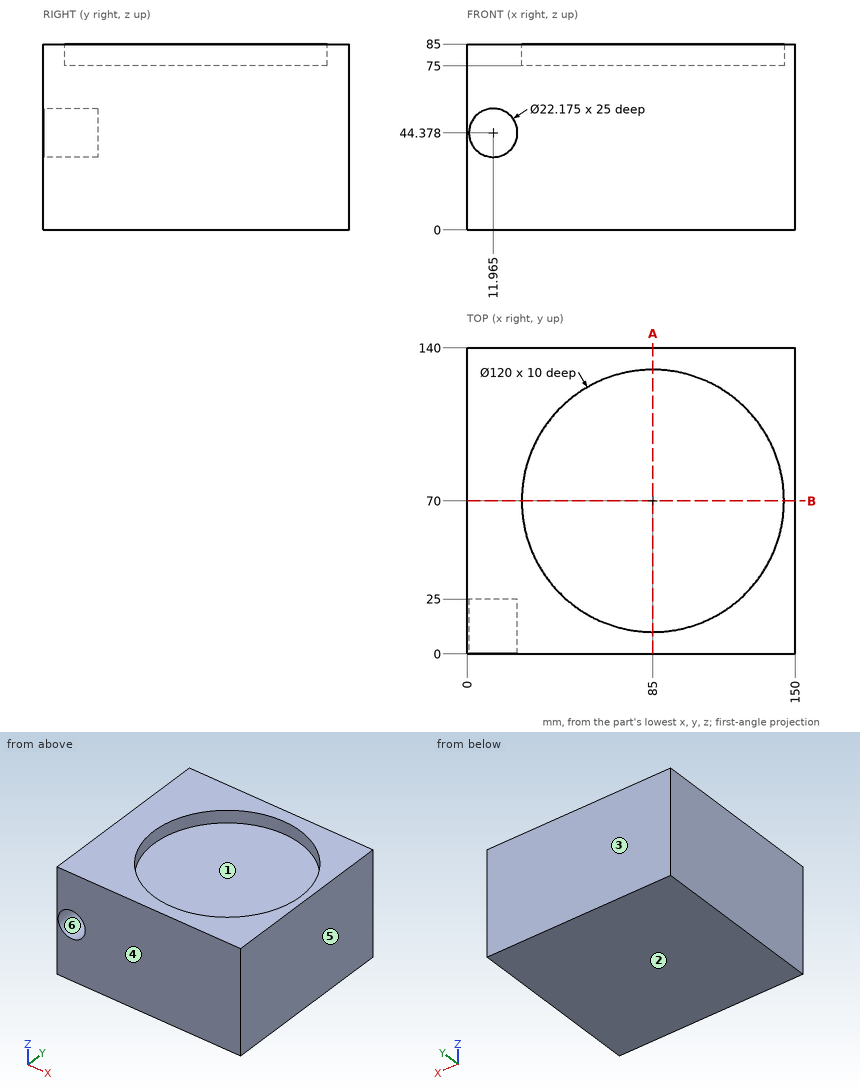
Here's the drawing with two shaded views (mm, measured from the low corner). I have some questions. A direction names the side the tool comes from. Give positions to 0.01 mm unless a question says otherwise; leave off trailing zeros. Loops run counter-clockwise (first coordinate to the right, second up) from the corner with the lowest first, then second, coordinate; pieces in that order, holes last. Notation, with made-up numbers: (60.5, 82.25) - (116.5, 82.25) arc R33 ccw to (116.5, 114.25) - close; hole circle Ø5 at (-15, 83.25). An arc over 180 degrees is marked (long way). One line per item, written item: value.
(1) If we mould it in two halves opening along Y, with no side actions, what happens to the marked faces 1, 2, 3 and 4? For each: released by +Y, released by -Y, zero draft, split by the parting line, or undercut.
Verdict:
face 1: undercut
face 2: zero draft
face 3: released by +Y
face 4: released by -Y
(2) If we section it at A-A, the plane x = 85: List the corners of the cut face in (y, z) for me, plus the area to 3 significant figures.
Verdict:
outline: (0, 0) - (140, 0) - (140, 85) - (130, 85) - (130, 75) - (10, 75) - (10, 85) - (0, 85) - close
area: 10,700 mm^2
(3) If we section it at B-B, the plane y = 70: List the corners of the cut face in (x, z) for me, plus the area to 4 significant figures.
Verdict:
outline: (0, 0) - (150, 0) - (150, 85) - (145, 85) - (145, 75) - (25, 75) - (25, 85) - (0, 85) - close
area: 11,550 mm^2
(4) On a 3-axis mill with a long thin cutter (end or side, diameter ignored), from which of +Z, -Z, +X, -X, +Y, -Y can I reach the whole of each face in a straight line? I mean the marked faces 5 and 6. Say none if no direction works.
Verdict:
face 5: +Z, -Z, +X, +Y, -Y
face 6: -Y
(5) I need wall thicknesses on line 1 along Y through (x, z) = (85, 80); line 2 along Z through (x, y) = (120, 69.5). Which ranges of each line are inside material? Lowest first, please.
Verdict:
line 1: 0 to 10, 130 to 140
line 2: 0 to 75
(6) I'm going to push a flat-ended pin straight in: pin 1 (1.5 mm diameter, centred on x = 46, y = 43.5, fed in from +Z). Where does the tip first touch, or does it pass through?
Verdict:
pin 1: z = 75
